Autodesk Inventor part; units mm, degrees
ref_plane "Plano de trabalho1" through (0, 0, -6) normal (0, 0, 1) x (1, 0, 0)
ref_plane "Plano de trabalho2" through (0, 0, 6) normal (0, 0, 1) x (1, 0, 0)
ref_plane "YZ Plane" through (0, 0, 0) normal (1, 0, 0) x (0, 1, 0)
sketch "Esboço1" plane through (0, 0, 0) normal (0, 1, 0) x (-1, 0, 0)
  circle A0 centre (0, 0) radius 6
  dimension "d0" = 12
extrude "Extrusão1" add sketch "Esboço1" along normal blind 90
chamfer "Chanfro1" distance 0.5 angle 45 1 edges at (6, 90, 0) measured on face at (0.7092, 90, 1.4219)
chamfer "Chanfro2" distance 0.5 angle 45 1 edges at (6, 0, 0) measured on face at (0.7092, 0, 1.4219)
ref_plane "Plano de trabalho1" through (0, 0, -6) normal (0, 0, 1) x (1, 0, 0)
ref_plane "Plano de trabalho2" through (0, 0, 6) normal (0, 0, 1) x (1, 0, 0)
sketch "Esboço2" plane through (0, 0, 6) normal (0, 0, 1) x (1, 0, 0)
  line L0 (6, 89.5) -> (-6, 89.5) construction
  line L1 (6, 89.5) -> (6, 61.5) construction
  line L2 (6, 0.5) -> (6, 89.5) construction
  line L3 (6, 61.5) -> (6, 51.5) construction
  line L4 (6, 0.5) -> (6, 12.5) construction
  line L5 (0, 61.5) -> (0, 51.5) construction
  line L6 (-1.25, 61.5) -> (-1.25, 51.5)
  line L7 (1.25, 51.5) -> (1.25, 61.5)
  arc A0 (1.25, 61.5) -> (-1.25, 61.5) centre (0, 61.5) ccw
  arc A1 (-1.25, 51.5) -> (1.25, 51.5) centre (0, 51.5) ccw
  line L8 (0, 12.5) -> (0, 0.5) construction
  line L9 (-6, 0.5) -> (6, 0.5)
  line L10 (-1.25, 12.5) -> (-1.25, 0.5)
  line L11 (1.25, 0.5) -> (1.25, 12.5)
  arc A2 (1.25, 12.5) -> (-1.25, 12.5) centre (0, 12.5) ccw
  arc A3 (-1.25, 0.5) -> (1.25, 0.5) centre (0, 0.5) ccw
  point P0 (0, 0)
  point P1 (0, 56.5)
  point P2 (0, 6.5)
  dimension "d9" = 28
  dimension "d10" = 10
  dimension "d11" = 12
  dimension "d12" = 2.5
  dimension "d13" = 2.5
extrude "Extrusão2" cut sketch "Esboço2" against normal blind 2.5 contours A0 L7 A1 L6 | L10 A2 L11 L9
properties part number "eixo 5"
For this review, take the finished solid that the model builds, in its own axes (mm). A direction names the side the tool comes from. Coordinates: 2 decimals unless noted, no trailing zeros. Loops run counter-clockwise (first coordinate to the right, second up) from the corner with the lowest first, then second, coordinate; pieces in that order, holes last. Notation, with made-up numbers: (-25, 89) - (10, 89) arc R19 cw to (10, 113) - close; hole circle Ø6 at (-28, 26). An arc over 180 degrees is marked (long way). Return JSON: item names as keys, results as strings.
Item 1: For line 1 (Z direction, x = 0.25, y = 55.5); line 2 (X direction, y = 9, z = 5.25); line 3 (Z direction, x = -2.5, y = 70), list the stretches that pass through material, from the lowest coordinate up.
Determined:
{"line 1": "z = -5.99 to 3.5", "line 2": "x = -2.9 to -1.25, 1.25 to 2.9", "line 3": "z = -5.45 to 5.45"}
Item 2: For faces 4 (the flat face through (0, 0.5, 5)), 5 (the flat face through (0, 0, 0)), list the 3-axis set-ups (+Z, -Z, +X, -X, +Y, -Y) from which the entire face can be reached by the end or side of a thin tool; tool diameter is ignored.
Determined:
{"face 4": "+Z", "face 5": "+Z, -Z, +X, -X, -Y"}
Item 3: Take a section at D-D (y = 16.5). Give the boundary of the cut face in (x, z), then the cut area to 3 significant figures.
Determined:
{"outline": "circle Ø12 at (0, 0)", "area": "113 mm2"}
Item 4: Insertion check: pin 1 (3 mm diameter, centred on x = 3, y = 38.5, fed in from -Z); pin 2 (3 mm diameter, centred on x = 4.5, z = -2.5, fed in from -Y); pin 3 (1.2 mm diameter, centred on y = 57.5, z = 4.5, fed in from +X); pin 4 (2 mm diameter, centred on y = 65.5, z = -4.5, fed in from +X). Each pin has a flat end and moves straight along its axis. Give the tip position at first contact, or say it passes through.
Determined:
{"pin 1": "stops at z = -5.81", "pin 2": "stops at y = 0", "pin 3": "stops at x = 4.56", "pin 4": "stops at x = 4.87"}
Item 5: Take a section at B-B (y = 52.5). Give the boundary of the cut face in (x, z), then the cut area to 3 significant figures.
Determined:
{"outline": "(-1.25, 3.5) - (-1.25, 5.87) arc R6 ccw (long way) to (1.25, 5.87) - (1.25, 3.5) - close", "area": "107 mm2"}
Item 6: Mouldability with a two-part tool opening along X and no side actions: class faces 1 (the flat face through (-1.25, 7, 5)), 2 (the flat face through (0, 90, 0)), 3 (the cylindrical face through (6, 44, 0)) as pulls with the +X half, pulls with the -X half, needs draft (parallel to the pull), parting line crosses it, or undercut.
Determined:
{"face 1": "undercut", "face 2": "needs draft", "face 3": "parting line crosses it"}
Item 7: Take a section at C-C (z = 4.75). State how many separate pieces and enclosed holes the cut face has, then the cut area to 3 significant figures.
Determined:
{"separate pieces": "1", "enclosed holes": "2", "area": "597 mm2"}
Item 8: Take a section at A-A (x = 0). Give the boundary of the cut face in (y, z), then the cut area to 3 significant figures.
Determined:
{"outline": "(0, -5.5) - (0.5, -6) - (89.5, -6) - (90, -5.5) - (90, 5.5) - (89.5, 6) - (62.75, 6) - (62.75, 3.5) - (50.25, 3.5) - (50.25, 6) - (13.75, 6) - (13.75, 3.5) - (0.5, 3.5) - (0.5, 6) - (0, 5.5) - close", "area": "1,020 mm2"}
